Here's how the part is built. I have some questions about the finished solid (model axes, mm). A direction names the side the tool comes from. Give positions to 0.01 mm unless a question says otherwise; leave off trailing zeros. Order: outer loops, then holes, each group sorted by start corner. A loop starts at its lowest first (then second) coordinate and runs counter-clockwise, first axis right, second up. Notation, with made-up numbers: M -27.5,-32.75 L -5.5,-32.75 A13 ccw -5.5,-28.75 Z; hole C 5.25,69.5 d1. An arc over 180 degrees is marked long. Use one line per item in the form item = value.
Solid Edge part; units mm, degrees
sketch "Sketch1" plane through (0, 0, 0) normal (0, 0, 1) x (1, 0, 0)
  line L0 (95, 16) -> (-95, 16)
  line L1 (-95, 16) -> (-95, -16)
  line L2 (-95, -16) -> (95, -16)
  line L3 (95, -16) -> (95, 16)
extrude "Protrusion1" add sketch "Sketch1" along normal mid plane 32
fillet "Round_1" radius 2 3 edges at (95, -16, 0) (-95, -16, 0) (-95, 16, 0)
sketch "Sketch2" plane through (0, 0, 16) normal (0, 0, 1) x (1, 0, 0)
  line L0 (67, 16) -> (92, 16)
  line L1 (92, 16) -> (92, 12)
  line L2 (92, 12) -> (67, 12)
  line L3 (67, 12) -> (67, 16)
extrude "ExtrudedCutout_1" cut sketch "Sketch2" against normal blind 60.1716
hole "Hole_3" at (-63, 0, 16) direction (0, 0, -1) diameter 12 depth 24 tip angle 118 countersink diameter 13 countersink angle 90
hole "Hole1" at (11, 0, 16) direction (0, 0, -1) diameter 12 depth 24 tip angle 118 countersink diameter 13 countersink angle 90
hole "Hole_6" at (-63, -16, 4) direction (0, 1, 0) diameter 4 depth 11.5 tip angle 118 countersink diameter 5 countersink angle 90
hole "Hole2" at (11, -16, 4) direction (0, 1, 0) diameter 4 depth 11.5 tip angle 118 countersink diameter 5 countersink angle 90
hole "Hole_8" at (77.5, -16, 4) direction (0, 1, 0) diameter 6.5 end through all countersink diameter 13 countersink angle 90
sketch "Sketch3" plane through (0, -16, 0) normal (0, -1, 0) x (1, 0, 0)
  circle A0 centre (-87, 6) radius 3
extrude "ExtrudedCutout_2" cut sketch "Sketch3" against normal blind 90
hole "Hole_9" at (-87, 0, 16) direction (0, 0, -1) diameter 1.5 depth 10 tip angle 118 countersink diameter 4 countersink angle 90
hole "Hole_10" at (-43, 0, 16) direction (0, 0, -1) diameter 4 depth 16 tip angle 118 countersink diameter 5 countersink angle 90
sketch "Sketch4" plane through (0, 0, 16) normal (0, 0, 1) x (1, 0, 0)
  circle A0 centre (-37, 10) radius 3
  circle A1 centre (37, 10) radius 3
extrude "ExtrudedCutout_3" cut sketch "Sketch4" against normal blind 60
Q1. I'm going to push flat-ended pins straight in: pin 1 Ø5 at (x, z) = (-87, 6) entering from -Y; pin 2 Ø2 at (x, y) = (-87, 0) entering from +Z; pin 3 Ø8.5 at (x, z) = (77.5, 4) entering from +Y. Where does each tip first touch, or does it pass through?
Found:
pin_1 = through
pin_2 = 15
pin_3 = 12
Q2. I want a section at A-A on y = 10. Write out the boundary of the cut face in (x, z).
Found:
outline = M -95,-16 L -40,-16 L -40,16 L -95,16 Z; M -34,-16 L 34,-16 L 34,16 L -34,16 Z; M 40,-16 L 95,-16 L 95,16 L 40,16 Z; hole C -87,6 d6; hole C 77.5,4 d6.5
Q3. Thinking about a two-plate mould opening in Z: for faces 1 (the face through (-43.34, 0.08, -0.99)), 2 (the face through (-95, 0, 0)), 3 (the face through (81, -13, 4)), which applies, +Z half, -Z half, draft (parallel to the pull), parting line (faces both ways), or undercut?
Found:
face_1 = +Z half
face_2 = draft
face_3 = undercut
Q4. I want a section at C-C on z = -6. Write out the boundary of the cut face in (x, y), then the cut area to 3 significant figures.
Found:
outline = M -95,-14 A2 ccw -93,-16 L 93,-16 A2 ccw 95,-14 L 95,16 L 92,16 L 92,12 L 67,12 L 67,16 L -93,16 A2 ccw -95,14 Z; hole C -63,0 d12; hole C -37,10 d6; hole C 11,0 d12; hole C 37,10 d6
area = 5,690 mm²
Q5. I want a section at B-B on x = 37. Write out the boundary of the cut face in (y, z), then the cut area to 3 significant figures.
Found:
outline = M -16,-16 L 7,-16 L 7,16 L -16,16 Z; M 13,-16 L 16,-16 L 16,16 L 13,16 Z
area = 832 mm²
Q6. I need wall thicknesses on L1, parallel to X at y = 0, z = 10.25; L2, parallel to Y at x = -37, z = 8; L3, parallel to X at y = 8.5, z = -11.5. Which ranges of each line are inside material? Lowest first, please.
Found:
L1 = -95 to -87.75, -86.25 to -69, -57 to -45, -41 to 5, 17 to 95
L2 = -16 to 7, 13 to 16
L3 = -95 to -39.6, -34.4 to 34.4, 39.6 to 95
Q7. On a 3-axis mill with a long thin cutter (end or side, diameter ignored), from which of +Z, -Z, +X, -X, +Y, -Y can I reach the whole of each face in a straight line? I mean faces 4 (the face through (92, 14, 0)), 5 (the face through (-1, -16, 0)), 6 (the face through (-59.35, 4.76, 3.59)). Say none if no direction works.
Found:
face_4 = +Z, -Z, +Y
face_5 = +Z, -Z, +X, -X, -Y
face_6 = +Z
Q8. I want a section at D-D on x = 77.5. Write out the boundary of the cut face in (y, z), then the cut area to 3 significant figures.
Found:
outline = M -16,-16 L 12,-16 L 12,0.75 L -12.75,0.75 L -16,-2.5 Z; M -16,10.5 L -12.75,7.25 L 12,7.25 L 12,16 L -16,16 Z
area = 703 mm²
